Verification items for the finished model (mm, model axes). A direction names the side the tool comes from. Give positions to 0.01 mm unless a question says otherwise; leave off trailing zeros. Loops run counter-clockwise (first coordinate to the right, second up) from the corner with the lowest first, then second, coordinate; pieces in that order, holes last. Notation, with made-up numbers: (12, 5.25) - (25, 5.25) arc R28 cw to (25, 34.25) - close; hole circle Ø10 at (-2.75, 41.25). An arc over 180 degrees is marked (long way). One line per item, written item: value. Start each with the question number.
1. Sectioned sample at B-B (x = -0.3). Record the cut outline in (y, z).
2. Sectioned sample at C-C (y = 3.5). Record the cut outline in (x, z) (3 decimals).
3. Sectioned sample at D-D (y = 17.5). Record the cut outline in (x, z) (3 decimals).
4. Access from +Z, -Z, +X, -X, +Y, -Y to the whole of each face (thin tool, end or side, straight path). Record for faces 1 (the cylindrical face through (0.046, 16.762, -2.525)), 2 (the flat face through (0, 0, 0)), 3 (the cylindrical face through (-0.046, 16.762, 2.525)).
5. Scan lines: L1, parallel to Y at x = 1.3, z = 0; L2, parallel to Z at x = 0.15, y = 3.5; L3, parallel to Z at x = 1.3, y = 3.5. Record each from-to range of solid material in increasing order. Write a range as [from, to].
6. Gauge pin test, flat end, axial feed: pin 1 (1.5 mm diameter, centred on y = 7.5, z = 3, fed in from -X). Record the tip position at first contact, or that the pin passes through.
7. Sectioned sample at A-A (z = 0). Record the cut outline in (x, y) (3 decimals), plus the area to 3 significant figures.
from build123d import *

# Parameters (mm, degrees)
SKETCH1_R               = 2.525
BOSS_EXTRUDE1_DEPTH     = 48
SKETCH2_R               = 6.1
BOSS_EXTRUDE2_DEPTH     = 14
SKETCH3_R               = 1.8
CUT_EXTRUDE1_DEPTH      = 7.1
CUT_EXTRUDE1_DEPTH_BACK = 7.1
SKETCH4_OUTSIDE_W       = 24.402
SKETCH4_OUTSIDE_H       = 24.402
SKETCH4_OUTSIDE_W_2     = 4.85
SKETCH4_OUTSIDE_H_2     = 23.377611606
CUT_EXTRUDE4_DEPTH      = 49


with BuildPart() as part:
    # Sketch1 → Boss-Extrude1 (new body)
    with BuildSketch(Plane(origin=(0, 0, 0), x_dir=(1, 0, 0), z_dir=(0, 1, 0))):
        Circle(SKETCH1_R)
    extrude(amount=BOSS_EXTRUDE1_DEPTH)

    # Sketch2 → Boss-Extrude2 (add)
    with BuildSketch(Plane(origin=(0, 48, 0), x_dir=(1, 0, 0), z_dir=(0, 1, 0))):
        Circle(SKETCH2_R)
    extrude(amount=-BOSS_EXTRUDE2_DEPTH)

    # Sketch3 → Cut-Extrude1 (cut, two sides)
    with BuildSketch(Plane(origin=(0, 0, 0), x_dir=(0, 0, -1), z_dir=(1, 0, 0))) as cut_extrude1_sk:
        with Locations((0, 3.5)):
            Circle(SKETCH3_R)
    extrude(amount=CUT_EXTRUDE1_DEPTH, mode=Mode.SUBTRACT)
    extrude(cut_extrude1_sk.sketch, amount=-CUT_EXTRUDE1_DEPTH_BACK, mode=Mode.SUBTRACT)

    # Sketch4 outside → Cut-Extrude4 (cut, through all)
    with BuildSketch(Plane(origin=(0, 0, 0), x_dir=(1, 0, 0), z_dir=(0, 1, 0))):
        Rectangle(SKETCH4_OUTSIDE_W, SKETCH4_OUTSIDE_H)
        Rectangle(SKETCH4_OUTSIDE_W_2, SKETCH4_OUTSIDE_H_2, mode=Mode.SUBTRACT)
    extrude(amount=CUT_EXTRUDE4_DEPTH, mode=Mode.SUBTRACT)


solid = part.part
Results are:
1. outline: (0, -2.51) - (34, -2.51) - (34, -6.09) - (48, -6.09) - (48, 6.09) - (34, 6.09) - (34, 2.51) - (0, 2.51) - close; hole circle Ø3.6 at (3.5, 0)
2. outline: (-1.771, -1.8) arc R2.525 ccw to (1.771, -1.8) - close; (-1.771, 1.8) - (1.771, 1.8) arc R2.525 ccw to start
3. outline: (-2.425, -0.704) arc R2.525 ccw to (2.425, -0.704) - (2.425, 0.704) arc R2.525 ccw to (-2.425, 0.704) - close
4. face 1: -Z, -Y
4. face 2: +Z, -Z, +X, -X, -Y
4. face 3: +Z, -Y
5. L1: y = [0, 1.7], [5.3, 48]
5. L2: z = [-2.52, -1.8], [1.8, 2.52]
5. L3: z = [-2.16, -1.8], [1.8, 2.16]
6. pin 1: stops at x = -1.15
7. outline: (-2.425, 0) - (2.425, 0) - (2.425, 1.7) - (-2.425, 1.7) - close; (-2.425, 5.3) - (2.425, 5.3) - (2.425, 48) - (-2.425, 48) - close
7. area: 215 mm^2
